Geometry check sheet. Reference: the model listing, model coordinates, mm. Face numbers are marked on the shaded views. Give positions to 0.01 mm unless a question says otherwise; leave off trailing zeros. Loops run counter-clockwise (first coordinate to the right, second up) from the corner with the lowest first, then second, coordinate; pieces in that order, holes last.
1. Cross-section at A-A, the plane z = -85. Record the cut outline in (x, y).
2. Release check for a two-part mould opening along Z. For the marked faces 1 and 2 record: +Z half, -Z half, draft (parallel to the pull), parting line (faces both ways), or undercut.
3. Material ranges on L1, parallel to X at y = 0.5, z = -85; L2, parallel to X at y = 8, z = 71; L3, parallel to Z at x = 43.5, y = 15.75, recorded low to high.
4. Cross-section at C-C, the plane x = 57.5. Record the cut outline in (y, z), plus the area to 3 significant figures.
5. Cross-section at D-D, the plane z = -38. Record the cut outline in (x, y).
6. Go/stop test with flat-tipped pins: pin 1 Ø22 at (x, z) = (-14.5, -66) entering from +Y; pin 2 Ø1.5 at (x, z) = (-70.5, 49) entering from +Y. Record where each tip stops, or that it passes through.
7. Cross-section at B-B, the plane y = 6.5. Record the cut outline in (x, z).
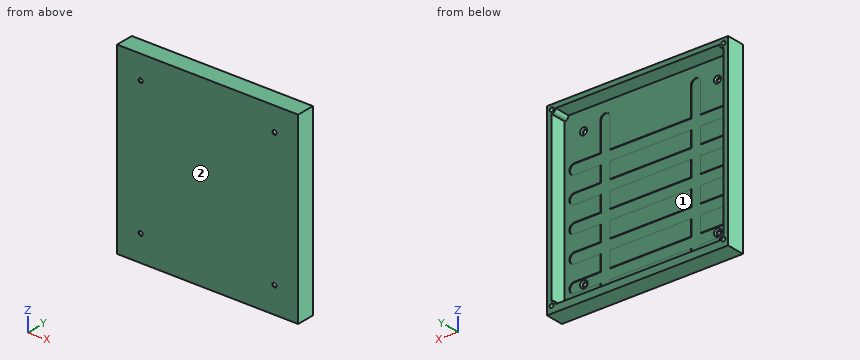
from build123d import *

# Parameters (mm, degrees)
CROQUIS1_W                                   = 230
CROQUIS1_H                                   = 233
CROQUIS1_R                                   = 2.65
SALIENTE_EXTRUIR1_DEPTH                      = 3
REFRENTADO_PARA_TORNILLO_TAP_N_CON_C_2_COUNT = 2
REFRENTADO_PARA_TORNILLO_TAP_N_CON_C_2_PITCH = 170
REFRENTADO_PARA_TORNILLO_TAP_N_CON_C_3_COUNT = 2
REFRENTADO_PARA_TORNILLO_TAP_N_CON_C_3_PITCH = 170
REFRENTADO_PARA_TORNILLO_TAP_N_CON_C_4_COUNT = 2
REFRENTADO_PARA_TORNILLO_TAP_N_CON_C_4_PITCH = 240.416305603
CROQUIS4_W                                   = 218.200156166
CROQUIS4_H                                   = 218.200156166
SALIENTE_EXTRUIR2_DEPTH                      = 20
CROQUIS5_R                                   = 5
SALIENTE_EXTRUIR3_DEPTH                      = 20
CROQUIS6_R                                   = 2.5
CORTAR_EXTRUIR1_DEPTH                        = 20
CORTAR_EXTRUIR2_DEPTH                        = 1
CORTAR_EXTRUIR3_START                        = -1
CORTAR_EXTRUIR3_OUTLINE_R                    = 4.48
CORTAR_EXTRUIR3_OUTLINE_W                    = 103
CORTAR_EXTRUIR3_OUTLINE_H                    = 13.137529202
CORTAR_EXTRUIR3_OUTLINE_H_2                  = 13.137529203
CORTAR_EXTRUIR3_DEPTH                        = 1


# Read off the part's stored shape, not the designer's step: Cortar-Extruir3
with BuildPart() as part:
    # Croquis1 → Saliente-Extruir1 (new body)
    with BuildSketch(Plane(origin=(0, 0, 0), x_dir=(1, 0, 0), z_dir=(0, 1, 0))):
        with Locations((0, 1.5)):
            Rectangle(CROQUIS1_W, CROQUIS1_H)
        with Locations(Location((-85, 85, 0), (0, 0, 270))):
            Circle(CROQUIS1_R, mode=Mode.SUBTRACT)
        with Locations(Location((-85, -85, 0), (0, 0, 270))):
            Circle(CROQUIS1_R, mode=Mode.SUBTRACT)
        with Locations(Location((85, -85, 0), (0, 0, 270))):
            Circle(CROQUIS1_R, mode=Mode.SUBTRACT)
        with Locations(Location((85, 85, 0), (0, 0, 270))):
            Circle(CROQUIS1_R, mode=Mode.SUBTRACT)
    extrude(amount=SALIENTE_EXTRUIR1_DEPTH)

    # Croquis3 → Refrentado para tornillo tapón con cabeza plana de clavija de M41 (revolve, cut)
    with BuildSketch(Plane(origin=(-85, 3, -85), x_dir=(0, 0, 1), z_dir=(1, 0, 0))):
        Polygon((0, 0), (0, 3), (2.25, 3), (2.25, 2.23), (4.48, 0), align=None)
    refrentado_para_tornillo_tap_n_con_cabez = revolve(axis=Axis((-85, 9.35, -85), (0, -1, 0)), mode=Mode.SUBTRACT)

    # Refrentado para tornillo tap_n con c 2: Refrentado para tornillo tapón con cabeza plana de clavija de M41 ×2
    with Locations(*[(i * REFRENTADO_PARA_TORNILLO_TAP_N_CON_C_2_PITCH, 0, 0) for i in range(1, REFRENTADO_PARA_TORNILLO_TAP_N_CON_C_2_COUNT)]):
        add(refrentado_para_tornillo_tap_n_con_cabez, mode=Mode.SUBTRACT)

    # Refrentado para tornillo tap_n con c 3: Refrentado para tornillo tapón con cabeza plana de clavija de M41 ×2
    with Locations(*[(0, 0, i * REFRENTADO_PARA_TORNILLO_TAP_N_CON_C_3_PITCH) for i in range(1, REFRENTADO_PARA_TORNILLO_TAP_N_CON_C_3_COUNT)]):
        add(refrentado_para_tornillo_tap_n_con_cabez, mode=Mode.SUBTRACT)

    # Refrentado para tornillo tap_n con c 4: Refrentado para tornillo tapón con cabeza plana de clavija de M41 ×2
    with Locations(*[Vector(0.7071067811865476, 0, 0.7071067811865475) * (i * REFRENTADO_PARA_TORNILLO_TAP_N_CON_C_4_PITCH) for i in range(1, REFRENTADO_PARA_TORNILLO_TAP_N_CON_C_4_COUNT)]):
        add(refrentado_para_tornillo_tap_n_con_cabez, mode=Mode.SUBTRACT)

    # Croquis4 → Saliente-Extruir2 (add)
    with BuildSketch(Plane(origin=(0, 3, 0), x_dir=(1, 0, 0), z_dir=(0, 1, 0))):
        Polygon((-115, 115), (-115, -115), (115, -115), (115, 115), (115, 118), (-115, 118), align=None)
        Rectangle(CROQUIS4_W, CROQUIS4_H, mode=Mode.SUBTRACT)
    extrude(amount=SALIENTE_EXTRUIR2_DEPTH)

    # Croquis5 → Saliente-Extruir3 (add)
    with BuildSketch(Plane(origin=(0, 23, 0), x_dir=(1, 0, 0), z_dir=(0, 1, 0))):
        with Locations((-109.100078083, 109.100078083)):
            Circle(CROQUIS5_R)
        with Locations((109.100078083, 109.100078083)):
            Circle(CROQUIS5_R)
        with Locations((109.100078083, -109.100078083)):
            Circle(CROQUIS5_R)
        with Locations((-109.100078083, -109.100078083)):
            Circle(CROQUIS5_R)
    extrude(amount=-SALIENTE_EXTRUIR3_DEPTH)

    # Croquis6 → Cortar-Extruir1 (cut)
    with BuildSketch(Plane(origin=(0, 23, 0), x_dir=(1, 0, 0), z_dir=(0, 1, 0))):
        with Locations(Location((-109.100078083, 109.100078083, 0), (0, 0, 270))):
            Circle(CROQUIS6_R)
        with Locations(Location((109.100078083, 109.100078083, 0), (0, 0, 90))):
            Circle(CROQUIS6_R)
        with Locations(Location((109.100078083, -109.100078083, 0), (0, 0, 270))):
            Circle(CROQUIS6_R)
        with Locations(Location((-109.100078083, -109.100078083, 0), (0, 0, 90))):
            Circle(CROQUIS6_R)
    extrude(amount=-CORTAR_EXTRUIR1_DEPTH, mode=Mode.SUBTRACT)

    # Croquis8 → Cortar-Extruir2 (cut)
    with BuildSketch(Plane(origin=(0, 3, 0), x_dir=(1, 0, 0), z_dir=(0, 1, 0))):
        with BuildLine():
            Line((-51.5, 95.5), (-51.5, -90))
            ThreePointArc((-51.5, -90), (-57.5, -96), (-63.5, -90))
            Line((-63.5, -90), (-63.5, 95.5))
            ThreePointArc((-63.5, 95.5), (-57.5, 101.5), (-51.5, 95.5))
        make_face()
        with BuildLine():
            Line((51.5, 95.5), (51.5, -90))
            ThreePointArc((51.5, -90), (57.5, -96), (63.5, -90))
            Line((63.5, -90), (63.5, 95.5))
            ThreePointArc((63.5, 95.5), (57.5, 101.5), (51.5, 95.5))
        make_face()
    extrude(amount=-CORTAR_EXTRUIR2_DEPTH, mode=Mode.SUBTRACT)

    # Cortar-Extruir3 outline → Cortar-Extruir3 (cut)
    # profile 1 of 15: a face of its own
    with BuildSketch(Plane(origin=(0, 3, 0), x_dir=(1, 0, 0), z_dir=(0, 1, 0)).offset(CORTAR_EXTRUIR3_START)):
        with BuildLine():
            ThreePointArc((-95.500196079, -40.431229574), (-102.06896068, -46.999994175), (-95.500196079, -53.568758776))
            Line((-95.500196079, -53.568758776), (-63.5, -53.568758776))
            Line((-63.5, -53.568758776), (-63.5, -40.431229574))
            Line((-63.5, -40.431229574), (-95.500196079, -40.431229574))
        make_face()
    # profile 2 of 15: a face of its own
    with BuildSketch(Plane(origin=(0, 3, 0), x_dir=(1, 0, 0), z_dir=(0, 1, 0)).offset(CORTAR_EXTRUIR3_START)):
        with BuildLine():
            Line((-95.509999989, 78.431242715), (-63.5, 78.431235399))
            Line((-63.5, 78.431235399), (-63.5, 91.568764601))
            Line((-63.5, 91.568764601), (-95.509999989, 91.568757285))
            ThreePointArc((-95.509999989, 91.568757285), (-102.06896068, 85), (-95.509999989, 78.431242715))
        make_face()
        with Locations((-85, 85)):
            Circle(CORTAR_EXTRUIR3_OUTLINE_R, mode=Mode.SUBTRACT)
    # profile 3 of 15: a face of its own
    with BuildSketch(Plane(origin=(0, 3, 0), x_dir=(1, 0, 0), z_dir=(0, 1, 0)).offset(CORTAR_EXTRUIR3_START)):
        with BuildLine():
            Line((-95.509999989, 45.431244171), (-63.5, 45.431236855))
            Line((-63.5, 45.431236855), (-63.5, 58.568766057))
            Line((-63.5, 58.568766057), (-95.509999989, 58.568758741))
            ThreePointArc((-95.509999989, 58.568758741), (-102.06896068, 52.000001456), (-95.509999989, 45.431244171))
        make_face()
    # profile 4 of 15: a face of its own
    with BuildSketch(Plane(origin=(0, 3, 0), x_dir=(1, 0, 0), z_dir=(0, 1, 0)).offset(CORTAR_EXTRUIR3_START)):
        with BuildLine():
            Line((-95.509999989, 12.431245628), (-63.5, 12.431238311))
            Line((-63.5, 12.431238311), (-63.5, 25.568767514))
            Line((-63.5, 25.568767514), (-95.509999989, 25.568760198))
            ThreePointArc((-95.509999989, 25.568760198), (-102.06896068, 19.000002913), (-95.509999989, 12.431245628))
        make_face()
    # profile 5 of 15: a face of its own
    with BuildSketch(Plane(origin=(0, 3, 0), x_dir=(1, 0, 0), z_dir=(0, 1, 0)).offset(CORTAR_EXTRUIR3_START)):
        with BuildLine():
            Line((-95.509999989, -20.568752916), (-63.5, -20.568760232))
            Line((-63.5, -20.568760232), (-63.5, -7.43123103))
            Line((-63.5, -7.43123103), (-95.509999989, -7.431238346))
            ThreePointArc((-95.509999989, -7.431238346), (-102.06896068, -13.999995631), (-95.509999989, -20.568752916))
        make_face()
    # profile 6 of 15: a face of its own
    with BuildSketch(Plane(origin=(0, 3, 0), x_dir=(1, 0, 0), z_dir=(0, 1, 0)).offset(CORTAR_EXTRUIR3_START)):
        with Locations((0, -46.999994175)):
            Rectangle(CORTAR_EXTRUIR3_OUTLINE_W, CORTAR_EXTRUIR3_OUTLINE_H)
    # profile 7 of 15: a face of its own
    with BuildSketch(Plane(origin=(0, 3, 0), x_dir=(1, 0, 0), z_dir=(0, 1, 0)).offset(CORTAR_EXTRUIR3_START)):
        with Locations((0, -13.999995631)):
            Rectangle(CORTAR_EXTRUIR3_OUTLINE_W, CORTAR_EXTRUIR3_OUTLINE_H)
    # profile 8 of 15: a face of its own
    with BuildSketch(Plane(origin=(0, 3, 0), x_dir=(1, 0, 0), z_dir=(0, 1, 0)).offset(CORTAR_EXTRUIR3_START)):
        with Locations((0, 19.000002913)):
            Rectangle(CORTAR_EXTRUIR3_OUTLINE_W, CORTAR_EXTRUIR3_OUTLINE_H_2)
    # profile 9 of 15: a face of its own
    with BuildSketch(Plane(origin=(0, 3, 0), x_dir=(1, 0, 0), z_dir=(0, 1, 0)).offset(CORTAR_EXTRUIR3_START)):
        with Locations((0, 52.000001456)):
            Rectangle(CORTAR_EXTRUIR3_OUTLINE_W, CORTAR_EXTRUIR3_OUTLINE_H)
    # profile 10 of 15: a face of its own
    with BuildSketch(Plane(origin=(0, 3, 0), x_dir=(1, 0, 0), z_dir=(0, 1, 0)).offset(CORTAR_EXTRUIR3_START)):
        with Locations((0, 85)):
            Rectangle(CORTAR_EXTRUIR3_OUTLINE_W, CORTAR_EXTRUIR3_OUTLINE_H)
    # profile 11 of 15: a face of its own
    with BuildSketch(Plane(origin=(0, 3, 0), x_dir=(1, 0, 0), z_dir=(0, 1, 0)).offset(CORTAR_EXTRUIR3_START)):
        with BuildLine():
            Line((63.5, -40.431229574), (63.5, -53.568758776))
            Line((63.5, -53.568758776), (96.509803921, -53.568758776))
            ThreePointArc((96.509803921, -53.568758776), (103.078568522, -46.999994175), (96.509803921, -40.431229574))
            Line((96.509803921, -40.431229574), (63.5, -40.431229574))
        make_face()
    # profile 12 of 15: a face of its own
    with BuildSketch(Plane(origin=(0, 3, 0), x_dir=(1, 0, 0), z_dir=(0, 1, 0)).offset(CORTAR_EXTRUIR3_START)):
        with BuildLine():
            Line((63.5, 91.568764601), (63.5, 78.431235399))
            Line((63.5, 78.431235399), (96.50980391, 78.431242715))
            ThreePointArc((96.50980391, 78.431242715), (103.068764601, 85), (96.50980391, 91.568757285))
            Line((96.50980391, 91.568757285), (63.5, 91.568764601))
        make_face()
        with Locations((85, 85)):
            Circle(CORTAR_EXTRUIR3_OUTLINE_R, mode=Mode.SUBTRACT)
    # profile 13 of 15: a face of its own
    with BuildSketch(Plane(origin=(0, 3, 0), x_dir=(1, 0, 0), z_dir=(0, 1, 0)).offset(CORTAR_EXTRUIR3_START)):
        with BuildLine():
            Line((63.5, 58.568766057), (63.5, 45.431236855))
            Line((63.5, 45.431236855), (96.50980391, 45.431244171))
            ThreePointArc((96.50980391, 45.431244171), (103.068764601, 52.000001456), (96.50980391, 58.568758741))
            Line((96.50980391, 58.568758741), (63.5, 58.568766057))
        make_face()
    # profile 14 of 15: a face of its own
    with BuildSketch(Plane(origin=(0, 3, 0), x_dir=(1, 0, 0), z_dir=(0, 1, 0)).offset(CORTAR_EXTRUIR3_START)):
        with BuildLine():
            Line((63.5, 25.568767514), (63.5, 12.431238311))
            Line((63.5, 12.431238311), (96.50980391, 12.431245628))
            ThreePointArc((96.50980391, 12.431245628), (103.068764601, 19.000002913), (96.50980391, 25.568760198))
            Line((96.50980391, 25.568760198), (63.5, 25.568767514))
        make_face()
    # profile 15 of 15: a face of its own
    with BuildSketch(Plane(origin=(0, 3, 0), x_dir=(1, 0, 0), z_dir=(0, 1, 0)).offset(CORTAR_EXTRUIR3_START)):
        with BuildLine():
            Line((63.5, -7.43123103), (63.5, -20.568760232))
            Line((63.5, -20.568760232), (96.50980391, -20.568752916))
            ThreePointArc((96.50980391, -20.568752916), (103.068764601, -13.999995631), (96.50980391, -7.431238346))
            Line((96.50980391, -7.431238346), (63.5, -7.43123103))
        make_face()
    extrude(amount=CORTAR_EXTRUIR3_DEPTH, mode=Mode.SUBTRACT)


solid = part.part
Result:
1. outline: (-115, 0) - (-87.65, 0) - (-87.65, 1.17) - (-89.48, 3) - (-89.48, 2) - (-102.07, 2) - (-102.07, 3) - (-109.1, 3) - (-109.1, 23) - (-115, 23) - close; (-82.35, 0) - (82.35, 0) - (82.35, 1.17) - (80.52, 3) - (80.52, 2) - (-80.52, 2) - (-80.52, 3) - (-82.35, 1.17) - close; (87.65, 0) - (115, 0) - (115, 23) - (109.1, 23) - (109.1, 3) - (103.07, 3) - (103.07, 2) - (89.48, 2) - (89.48, 3) - (87.65, 1.17) - close
2. face 1: undercut
2. face 2: draft
3. L1: x = -115 to -87.65, -82.35 to 82.35, 87.65 to 115
3. L2: x = -115 to -109.1, 109.1 to 115
3. L3: z = -118 to -109.1, 109.1 to 115
4. outline: (0, -118) - (23, -118) - (23, -109.1) - (3, -109.1) - (3, -101.5) - (2, -101.5) - (2, 96) - (3, 96) - (3, 109.1) - (23, 109.1) - (23, 115) - (0, 115) - close
4. area: 797 mm2
5. outline: (-115, 0) - (115, 0) - (115, 23) - (109.1, 23) - (109.1, 3) - (63.5, 3) - (63.5, 2) - (51.5, 2) - (51.5, 3) - (-51.5, 3) - (-51.5, 2) - (-63.5, 2) - (-63.5, 3) - (-109.1, 3) - (-109.1, 23) - (-115, 23) - close
6. pin 1: stops at y = 3
6. pin 2: stops at y = 2
7. outline: (-115, -118) - (115, -118) - (115, 115) - (-115, 115) - close; hole circle Ø5 at (-109.1, -109.1); hole circle Ø5 at (-109.1, 109.1); hole (-109.1, -104.1) arc R5 cw to (-104.1, -109.1) - (104.1, -109.1) arc R5 cw to (109.1, -104.1) - (109.1, 104.1) arc R5 cw to (104.1, 109.1) - (-104.1, 109.1) arc R5 cw to (-109.1, 104.1) - close; hole circle Ø5 at (109.1, -109.1); hole circle Ø5 at (109.1, 109.1)
